The listing builds one solid part. Answer for the finished solid, in the listing's coordinates (mm). A direction names the side the tool comes from. Give positions to 0.01 mm unless a question says otherwise; leave off trailing zeros. Order: outer loops, then holes, each group sorted by start corner. A loop starts at its lowest first (then second) coordinate and runs counter-clockwise, first axis right, second up. Notation, with made-up numbers: (-30, 61) - (5, 61) arc R9 ccw to (5, 68) - close; hole circle Ø7 at (47, 48.25). An arc over 180 degrees is marked (long way). Answer as a JSON object with one key per item and string values. Group by question number.
Q1. The mould has two halves that part along X. Classify faces 3 (the face through (87, 49, -16)), 4 (the face through (98.4, 49.4, -47.3)), 5 (the face through (-104.086, 49.442, -24.45)), 6 (the face through (101.975, 49, -22)): released by +X, released by -X, zero draft, split by the parting line, or undercut.
Q2. A cutting plane is placed at B-B, the plane x = 74. Give the vertices of the cut face in (y, z), and give its area (3 significant figures).
Q3. A cutting plane is placed at C-C, the plane z = -22.5. Give the vertices of the cut face in (x, y).
Q4. A cutting plane is placed at A-A, the plane y = 50.25. Give the vertices of the cut face in (x, z), and give its area (3 significant figures).
Q5. For faces 1 (the face through (15, 52.4, -18)), 2 (the face through (91.047, 49.442, -45.949)), determine the directions among +Z, -Z, +X, -X, +Y, -Y from which every point of the face is accessible in a straight line to the end or side of a thin tool.
Q6. Given pin 1 (1.5 mm diameter, centred on y = 50, z = -47, fed in from +X); pin 2 (1.5 mm diameter, centred on x = -71, y = 48, fed in from +Z), each flat-ended and moving along its own axis, determine where each tip first touches the part or whether it passes through.
Q7. A cutting plane is placed at D-D, the plane x = -81.5. Give the vertices of the cut face in (y, z), and give its area (3 significant figures).
Q8. Consider line 1 (Z direction, x = 96, y = 50.05); line 2 (Z direction, x = -16, y = 50.9); line 3 (Z direction, x = -61, y = 48.7). Determine where each line is inside the solid, lowest interval first.
from build123d import *

# Parameters (mm, degrees)
EXTRUDE_THIN1_DEPTH = 3


with BuildPart() as part:
    # Sketch1 → Extrude-Thin1 (new, symmetric)
    with BuildSketch(Plane(origin=(0, 49.4, 0), x_dir=(1, 0, 0), z_dir=(0, 1, 0))):
        with BuildLine():
            Line((84.13477336, 49.209016257), (89.109258274, 49.713496032))
            Line((89.109258274, 49.713496032), (94.581141252, 45.941641467))
            ThreePointArc((94.581141252, 45.941641467), (98.421521165, 47.378521725), (95.747760112, 50.487242457))
            Line((95.747760112, 50.487242457), (-96.710506132, 30.969381896))
            ThreePointArc((-96.710506132, 30.969381896), (-102.09834696, 24.714771507), (-96.140865711, 19.000106419))
            Line((-96.140865711, 19.000106419), (71.775188242, 18))
            Line((71.775188242, 18), (99.975188242, 18))
            Line((99.975188242, 18), (99.975188242, 25.9))
            Line((99.975188242, 25.9), (53.816953341, 18.20696085))
            Line((53.816953341, 18.20696085), (48.816953341, 18.236740802))
            Line((48.816953341, 18.236740802), (48.82886511, 20.236705329))
            Line((48.82886511, 20.236705329), (53.65734488, 20.20794695))
            Line((53.65734488, 20.20794695), (101.975188242, 28.260920843))
            Line((101.975188242, 28.260920843), (101.975188242, 16))
            Line((101.975188242, 16), (71.769232304, 16))
            Line((71.769232304, 16), (-96.152777481, 17.000141892))
            ThreePointArc((-96.152777481, 17.000141892), (-104.096085812, 24.619695343), (-96.912298043, 32.959175862))
            Line((-96.912298043, 32.959175862), (95.545968202, 52.477036422))
            ThreePointArc((95.545968202, 52.477036422), (100.358738097, 46.881339105), (93.446054253, 44.29495464))
            Line((93.446054253, 44.29495464), (88.579542516, 47.649517336))
            Line((88.579542516, 47.649517336), (84.33656527, 47.219222292))
            Line((84.33656527, 47.219222292), (84.13477336, 49.209016257))
        make_face()
    extrude(amount=EXTRUDE_THIN1_DEPTH, both=True)


solid = part.part
Reply:
{
 "1": {"face 3": "zero draft", "face 4": "undercut", "face 5": "released by -X", "face 6": "released by +X"},
 "2": {"outline": "(46.4, -50.29) - (52.4, -50.29) - (52.4, -48.28) - (46.4, -48.28) - close; (46.4, -23.6) - (52.4, -23.6) - (52.4, -21.57) - (46.4, -21.57) - close; (46.4, -18) - (52.4, -18) - (52.4, -16) - (46.4, -16) - close", "area": "36.2 mm^2"},
 "3": {"outline": "(-103.7, 46.4) - (-101.56, 46.4) - (-101.56, 52.4) - (-103.7, 52.4) - close; (67.41, 46.4) - (79.58, 46.4) - (79.58, 52.4) - (67.41, 52.4) - close; (99.98, 46.4) - (101.98, 46.4) - (101.98, 52.4) - (99.98, 52.4) - close"},
 "4": {"outline": "(-96.91, -32.96) - (95.55, -52.48) arc R4.5 ccw (long way) to (93.45, -44.29) - (88.58, -47.65) - (84.34, -47.22) - (84.13, -49.21) - (89.11, -49.71) - (94.58, -45.94) arc R2.5 cw (long way) to (95.75, -50.49) - (-96.71, -30.97) arc R6 cw to (-96.14, -19) - (71.78, -18) - (99.98, -18) - (99.98, -25.9) - (53.82, -18.21) - (48.82, -18.24) - (48.83, -20.24) - (53.66, -20.21) - (101.98, -28.26) - (101.98, -16) - (71.77, -16) - (-96.15, -17) arc R8 ccw to start", "area": "998 mm^2"},
 "5": {"face 1": "+Z, -Z, +X, -X, +Y", "face 2": "+Y, -Y"},
 "6": {"pin 1": "stops at x = 100.49", "pin 2": "stops at z = -16.85"},
 "7": {"outline": "(46.4, -34.52) - (52.4, -34.52) - (52.4, -32.51) - (46.4, -32.51) - close; (46.4, -18.91) - (52.4, -18.91) - (52.4, -16.91) - (46.4, -16.91) - close", "area": "24.1 mm^2"},
 "8": {"line 1": "z = -52.5 to -50.5, -45.5 to -43.5, -27.27 to -25.24, -18 to -16", "line 2": "z = -41.16 to -39.15, -18.52 to -16.52", "line 3": "z = -36.6 to -34.59, -18.79 to -16.79"}
}
